from build123d import *

# Parameters (mm, degrees)
F0_W     = 30
F0_H     = 20
F1_DEPTH = 40
F2_W     = 26
F2_H     = 16
F3_DEPTH = 38
F4_W     = 27
F4_H     = 17
F5_DEPTH = 5
F6_R     = 3


with BuildPart() as f1:
    # F0 (on Top) → F1 (new body)
    with BuildSketch(Plane.XY):
        with Locations((-5.625001, 19.210285)):
            Rectangle(F0_W, F0_H)
    extrude(amount=F1_DEPTH)

    # F2 (on face) → F3 (cut)
    with BuildSketch(Plane.XY.offset(40)):
        with Locations((-5.625001, 19.210285)):
            Rectangle(F2_W, F2_H)
    extrude(amount=-F3_DEPTH, mode=Mode.SUBTRACT)

    # F4 (on face) → F5 (cut)
    with BuildSketch(Plane.XY.offset(40)):
        with Locations((-5.625001, 19.210285)):
            Rectangle(F4_W, F4_H)
    extrude(amount=-F5_DEPTH, mode=Mode.SUBTRACT)

    # F6
    f6_edges = [f1.edges().sort_by_distance(p)[0] for p in [
        (-20.625001, 9.210285, 20),
        (-20.625001, 29.210285, 20),
        (9.374999, 9.210285, 20),
        (9.374999, 29.210285, 20),
    ]]
    fillet(f6_edges, radius=F6_R)


solid = f1.part
Geometry: final body of the model. Coordinates: model frame, mm. A direction names the side the tool comes from. Round coordinates to 2 decimals unless told otherwise and drop trailing zeros. Loops run counter-clockwise (first coordinate to the right, second up) from the corner with the lowest first, then second, coordinate; pieces in that order, holes last.
Q1. Access query for faces 1 (the cylindrical face through (8.473, 10.066, 20.28)), 2 (the flat face through (-6, 27.21, 19)). Directions: +Z, -Z, +X, -X, +Y, -Y. A direction counts if a zero-diameter tool reaches every point of the face in a straight line with its end or side. Return the directions, or none.
Q2. Section A-A on z = 18.5. Return loops of the section in (x, y) (3 decimals).
Q3. Section B-B on x = -3. Return loops of the section in (y, z), plus the area to 3 significant figures.
Q4. Material intervals for L1, parallel to Y at x = -2.75, z = 3; L2, parallel to X at y = 16.25, z = 3 (3 decimals); L3, parallel to Y at x = -4, z = 37, sorted ascending.
Q5. Pull-direction query (X, two-part tool) for faces 3 (the flat face through (7.375, 19, 19)), 4 (the flat face through (9.375, 19, 20)), 5 (the flat face through (-20.625, 19, 20)); classes: released by +X, released by -X, zero draft, split by the parting line, or undercut.
Q6. Pin query (flat end, axial travel): P1, Ø1, axis at x = -5.5, y = 19.5, coming from the +Z side. Return the tip coordinate at first contact, or that it passes through.
Q7. Section C-C on y = 21. Return loops of the section in (x, z) (3 decimals), plus the area to 3 significant figures.
Evaluation:
1. face 1: +Z, -Z, +X, -Y
1. face 2: +Z
2. outline: (-20.625, 12.21) arc R3 ccw to (-17.625, 9.21) - (6.375, 9.21) arc R3 ccw to (9.375, 12.21) - (9.375, 26.21) arc R3 ccw to (6.375, 29.21) - (-17.625, 29.21) arc R3 ccw to (-20.625, 26.21) - close; hole (-18.625, 11.21) - (7.375, 11.21) - (7.375, 27.21) - (-18.625, 27.21) - close
3. outline: (9.21, 0) - (29.21, 0) - (29.21, 40) - (27.71, 40) - (27.71, 35) - (27.21, 35) - (27.21, 2) - (11.21, 2) - (11.21, 35) - (10.71, 35) - (10.71, 40) - (9.21, 40) - close
3. area: 187 mm2
4. L1: y = 9.21 to 11.21, 27.21 to 29.21
4. L2: x = -20.625 to -18.625, 7.375 to 9.375
4. L3: y = 9.21 to 10.71, 27.71 to 29.21
5. face 3: undercut
5. face 4: released by +X
5. face 5: released by -X
6. P1: stops at z = 2
7. outline: (-20.625, 0) - (9.375, 0) - (9.375, 40) - (7.875, 40) - (7.875, 35) - (7.375, 35) - (7.375, 2) - (-18.625, 2) - (-18.625, 35) - (-19.125, 35) - (-19.125, 40) - (-20.625, 40) - close
7. area: 207 mm2
